```python
from build123d import *

# Parameters (mm, degrees)
CYLINDER001_R         = 47
CYLINDER001_DEPTH     = 5
CYLINDER_R            = 40
CYLINDER_DEPTH        = 105
SKETCH_R              = 12.2
POCKET_DEPTH          = 100.001
SKETCH001_R           = 12.2
POCKET001_DEPTH       = 438.804778
POLARPATTERN_COUNT    = 6
SKETCH002_R           = 7
POCKET002_DEPTH       = 105.001
SKETCH003_R           = 7
POCKET003_DEPTH       = 443.804778
POLARPATTERN001_COUNT = 6
SKETCH004_R           = 38.7
POCKET004_DEPTH       = 4.001
SKETCH005_R           = 2
POCKET005_DEPTH       = 439.804778
POCKET005_DEPTH_BACK  = 342.804778
POLARPATTERN002_COUNT = 3
SKETCH006_R           = 1.5
POCKET006_DEPTH       = 338.804778
POCKET006_DEPTH_BACK  = 443.804778
POLARPATTERN003_COUNT = 4
SKETCH007_W           = 3.25
SKETCH007_H           = 6.5
POCKET007_DEPTH       = 338.804778
POCKET007_DEPTH_BACK  = 443.804778
POLARPATTERN004_COUNT = 3


with BuildPart() as obj1:
    # Cylinder001 → Cylinder001 (new body)
    with BuildSketch(Plane.XY.offset(20)):
        Circle(CYLINDER001_R)
    extrude(amount=CYLINDER001_DEPTH)


with BuildPart() as corps:
    # Cylinder → Cylinder (new body)
    with BuildSketch(Plane.XY):
        Circle(CYLINDER_R)
    extrude(amount=CYLINDER_DEPTH)

    # Fusion: union obj1
    add(obj1.part)

    # Sketch → Pocket (cut, through all)
    with BuildSketch(Plane.XY.offset(5)):
        Circle(SKETCH_R)
    extrude(amount=POCKET_DEPTH, mode=Mode.SUBTRACT)

    # Sketch001 → Pocket001 (cut, through all)
    with BuildSketch(Plane(origin=(26, 0, 5), x_dir=(1, 0, 0), z_dir=(0, 0, 1))):
        Circle(SKETCH001_R)
    pocket001 = extrude(amount=POCKET001_DEPTH, mode=Mode.SUBTRACT)

    # PolarPattern: Pocket001 ×6 about axis
    polarpattern_axis = Axis((0, 0, 0), (0, 0, 1))
    for i in range(1, POLARPATTERN_COUNT):
        add(pocket001.rotate(polarpattern_axis, i * 360 / POLARPATTERN_COUNT), mode=Mode.SUBTRACT)

    # Sketch002 → Pocket002 (cut, through all)
    with BuildSketch(Plane.XY):
        Circle(SKETCH002_R)
    extrude(amount=POCKET002_DEPTH, mode=Mode.SUBTRACT)

    # Sketch003 → Pocket003 (cut, through all)
    with BuildSketch(Plane(origin=(25, 0, 0), x_dir=(1, 0, 0), z_dir=(0, 0, 1))):
        Circle(SKETCH003_R)
    pocket003 = extrude(amount=POCKET003_DEPTH, mode=Mode.SUBTRACT)

    # PolarPattern001: Pocket003 ×6 about axis
    polarpattern001_axis = Axis((0, 0, 0), (0, 0, 1))
    for i in range(1, POLARPATTERN001_COUNT):
        add(pocket003.rotate(polarpattern001_axis, i * 360 / POLARPATTERN001_COUNT), mode=Mode.SUBTRACT)

    # Sketch004 → Pocket004 (cut, through all)
    with BuildSketch(Plane.XY.offset(101)):
        Circle(SKETCH004_R)
    extrude(amount=POCKET004_DEPTH, mode=Mode.SUBTRACT)

    # Sketch005 → Pocket005 (cut, two sides)
    with BuildSketch(Plane(origin=(0, -34, 101), x_dir=(1, 0, 0), z_dir=(0, 0, 1))) as pocket005_sk:
        Circle(SKETCH005_R)
    pocket005 = extrude(amount=-POCKET005_DEPTH, mode=Mode.SUBTRACT) + extrude(pocket005_sk.sketch, amount=POCKET005_DEPTH_BACK, mode=Mode.SUBTRACT)

    # PolarPattern002: Pocket005 ×3 about axis
    polarpattern002_axis = Axis((0, 0, 0), (0, 0, 1))
    for i in range(1, POLARPATTERN002_COUNT):
        add(pocket005.rotate(polarpattern002_axis, i * 360 / POLARPATTERN002_COUNT), mode=Mode.SUBTRACT)

    # Sketch006 → Pocket006 (cut, two sides)
    with BuildSketch(Plane(origin=(0, 43.5, 0), x_dir=(1, 0, 0), z_dir=(0, 0, 1))) as pocket006_sk:
        Circle(SKETCH006_R)
    pocket006 = extrude(amount=-POCKET006_DEPTH, mode=Mode.SUBTRACT) + extrude(pocket006_sk.sketch, amount=POCKET006_DEPTH_BACK, mode=Mode.SUBTRACT)

    # PolarPattern003: Pocket006 ×4 about axis
    polarpattern003_axis = Axis((0, 0, 0), (0, 0, 1))
    for i in range(1, POLARPATTERN003_COUNT):
        add(pocket006.rotate(polarpattern003_axis, i * 360 / POLARPATTERN003_COUNT), mode=Mode.SUBTRACT)

    # Sketch007 → Pocket007 (cut, two sides)
    with BuildSketch(Plane(origin=(0, 33, 0), x_dir=(1, 0, 0), z_dir=(0, 0, 1))) as pocket007_sk:
        Rectangle(SKETCH007_W, SKETCH007_H)
    pocket007 = extrude(amount=-POCKET007_DEPTH, mode=Mode.SUBTRACT) + extrude(pocket007_sk.sketch, amount=POCKET007_DEPTH_BACK, mode=Mode.SUBTRACT)

    # PolarPattern004: Pocket007 ×3 about axis
    polarpattern004_axis = Axis((0, 0, 0), (0, 0, 1))
    for i in range(1, POLARPATTERN004_COUNT):
        add(pocket007.rotate(polarpattern004_axis, i * 360 / POLARPATTERN004_COUNT), mode=Mode.SUBTRACT)


solid = corps.part
```
CAD build for the part. Positions are in the model's coordinates, mm. A direction names the side the tool comes from. Round coordinates to 2 decimals unless told otherwise and drop trailing zeros. Loops run counter-clockwise (first coordinate to the right, second up) from the corner with the lowest first, then second, coordinate; pieces in that order, holes last. Notation, with made-up numbers: M -13,-7 L 27,-7 A19 cw 27,27 Z; hole C 38,84.5 d1. An arc over 180 degrees is marked long. Return JSON: item names as keys, results as strings. Group by question number.
(1) Saw through at A-A, the plane x = -43.5. List the corners of the cut face in (y, z), and give its area (3 significant figures).
(2) Tool access for faces 1 (the cylindrical face through (-8.67, -39.05, 9.86)), 2 (the flat face through (-1.625, 33, 50)), 3 (the flat face through (-20, -24, 5)): list every direction of +Z, -Z, +X, -X, +Y, -Y with a clear straight run to the whole face (end or side of a thin tool).
(3) Drop flat-ended pins along their axis: P1, Ø22.5, axis at x = 12.5, y = -21.65, coming from the -Z side; P2, Ø1, axis at x = -30.5, z = 83, coming from the -Y side; P3, Ø2, axis at y = 17, z = 62, coming from the -X side; P4, Ø12, axis at x = -8, y = -23, coming from the +Z side. Give the stop position or say it passes through.
(4) Wall check: probe 1 along X at (y, z) = (-19, 81); probe 2 along X at (y, z) = (-6, 63); probe 3 along Y at (x, z) = (-7.5, 99). Give the ranges that are in metal, low to high. Write a range as [from, to].
(5) Saw through at B-B, the plane z = 83.5. Give the number of separate pieces and of enclosed holes in the cut face, and give its area (3 significant figures).
(6) Mould opens along Y. For faces 4 (the cylindrical face through (-8.67, -39.05, 64.44)), 5 (the flat face through (-25.753, -14.895, 51.207)) say: +Y half, -Y half, draft (parallel to the pull), parting line (faces both ways), or undercut.
Answer list:
{
 "1": {"outline": "M -17.8,20 L -1.5,20 L -1.5,25 L -17.8,25 Z; M 1.5,20 L 17.8,20 L 17.8,25 L 1.5,25 Z", "area": "163 mm2"},
 "2": {"face 1": "-Z", "face 2": "+Z, -Z", "face 3": "+Z"},
 "3": {"P1": "z = 0", "P2": "y = -26.46", "P3": "x = -36.66", "P4": "z = 5"},
 "4": {"probe 1": "[-35.2, -30.89], [-29.66, -24.68], [-1.32, 1.32], [24.68, 29.66], [30.89, 35.2]", "probe 2": "[-39.55, -36.62], [-15.38, -10.62], [10.62, 15.38], [36.62, 39.55]", "probe 3": "[-39.29, -33.41], [-11.63, -9.62], [9.62, 11.63], [33.41, 39.29]"},
 "5": {"separate pieces": "1", "enclosed holes": "13", "area": "1,650 mm2"},
 "6": {"face 4": "parting line", "face 5": "undercut"}
}
